```python
from build123d import *

# Parameters (mm, degrees)
F0_W      = 23
F0_H      = 16
F1_DEPTH  = 21
F2_R      = 2.5
F3_W      = 9.25
F3_H      = 5.75
F4_DEPTH  = 18
F5_R      = 1.5
F6_W      = 2
F6_H      = 12
F7_DEPTH  = 1.5
F8_W      = 2
F8_H      = 12
F9_DEPTH  = 1.5
F10_W     = 2
F10_H     = 12
F11_DEPTH = 1.5
F14_DEPTH = 3.5
F16_DEPTH = 1
F18_W     = 7.25
F18_H     = 1.5
F17_W     = 7.25
F17_H     = 1.5
F19_DEPTH = 0.5
F20_R     = 1.5
F21_DEPTH = 13


with BuildPart() as f1:
    # F0 (on Top) → F1 (new body)
    with BuildSketch(Plane.XY):
        Rectangle(F0_W, F0_H)
    extrude(amount=-F1_DEPTH)

    # F2
    f2_edges = [f1.edges().sort_by_distance(p)[0] for p in [
        (11.5, -8, -10.5),
        (11.5, 8, -10.5),
        (-11.5, -8, -10.5),
        (-11.5, 8, -10.5),
    ]]
    fillet(f2_edges, radius=F2_R)

    # F3 (on face) → F4 (cut)
    with BuildSketch(Plane.XY):
        with Locations((-5.375, 3.625)):
            Rectangle(F3_W, F3_H)
        with Locations((5.375, 3.625)):
            Rectangle(F3_W, F3_H)
        with Locations((5.375, -3.625)):
            Rectangle(F3_W, F3_H)
        with Locations((-5.375, -3.625)):
            Rectangle(F3_W, F3_H)
    extrude(amount=-F4_DEPTH, mode=Mode.SUBTRACT)

    # F5
    f5_edges = [f1.edges().sort_by_distance(p)[0] for p in [
        (-10, 6.5, -9),
        (-10, -6.5, -9),
        (10, -6.5, -9),
        (10, 6.5, -9),
    ]]
    fillet(f5_edges, radius=F5_R)

    # F6 (on face) → F7 (cut, through all)
    with BuildSketch(Plane.YZ.offset(0.75)):
        with Locations((-5.5, -6)):
            Rectangle(F6_W, F6_H)
        with Locations((5.5, -6)):
            Rectangle(F6_W, F6_H)
    extrude(amount=-F7_DEPTH, mode=Mode.SUBTRACT)

    # F8 (on face) + F7_face (on face) → F9 (cut, through all)
    with BuildSketch(Plane(origin=(0, 8, 0), x_dir=(-1, 0, 0), z_dir=(0, 1, 0))):
        with Locations((7.5, -6)):
            Rectangle(F8_W, F8_H)
        with Locations((-7.5, -6)):
            Rectangle(F8_W, F8_H)
    with BuildSketch(Plane(origin=(0, 6.5, -8.8181818182), x_dir=(1, 0, 0), z_dir=(0, -1, 0))):
        Polygon((8.5, 8.8181818182), (-8.5, 8.8181818182), (-8.5, -9.1818181818), (-0.75, -9.1818181818), (-0.75, -3.1818181818), (0.75, -3.1818181818), (0.75, -9.1818181818), (8.5, -9.1818181818), align=None)
    extrude(amount=-F9_DEPTH, dir=(0, 1, 0), mode=Mode.SUBTRACT)

    # F10 (on face) → F11 (cut, through all)
    with BuildSketch(Plane.XZ.offset(8)):
        with Locations((-7.5, -6)):
            Rectangle(F10_W, F10_H)
        with Locations((7.5, -6)):
            Rectangle(F10_W, F10_H)
    extrude(amount=-F11_DEPTH, mode=Mode.SUBTRACT)

    # F13 (on face) → F14 (join)
    with BuildSketch(Plane.XY):
        with BuildLine():
            Line((-11.5, 5), (-10, 5))
            ThreePointArc((-10, 5), (-9.5606601718, 6.0606601718), (-8.5, 6.5))
            Line((-8.5, 6.5), (-8.5, 8))
            Line((-8.5, 8), (-9, 8))
            ThreePointArc((-9, 8), (-10.767766953, 7.267766953), (-11.5, 5.5))
            Line((-11.5, 5.5), (-11.5, 5))
        make_face()
        with BuildLine():
            Line((-10, -5), (-11.5, -5))
            Line((-11.5, -5), (-11.5, -5.5))
            ThreePointArc((-11.5, -5.5), (-10.767766953, -7.267766953), (-9, -8))
            Line((-9, -8), (-8.5, -8))
            Line((-8.5, -8), (-8.5, -6.5))
            ThreePointArc((-8.5, -6.5), (-9.5606601718, -6.0606601718), (-10, -5))
        make_face()
        with BuildLine():
            Line((11.5, -5), (10, -5))
            ThreePointArc((10, -5), (9.5606601718, -6.0606601718), (8.5, -6.5))
            Line((8.5, -6.5), (8.5, -8))
            Line((8.5, -8), (9, -8))
            ThreePointArc((9, -8), (10.767766953, -7.267766953), (11.5, -5.5))
            Line((11.5, -5.5), (11.5, -5))
        make_face()
        with BuildLine():
            ThreePointArc((8.5, 6.5), (9.5606601718, 6.0606601718), (10, 5))
            Line((10, 5), (11.5, 5))
            Line((11.5, 5), (11.5, 5.5))
            ThreePointArc((11.5, 5.5), (10.767766953, 7.267766953), (9, 8))
            Line((9, 8), (8.5, 8))
            Line((8.5, 8), (8.5, 6.5))
        make_face()
    extrude(amount=F14_DEPTH)

    # F15 (on face) → F16 (join)
    with BuildSketch(Plane.XY):
        Polygon((-0.75, 0.75), (-2.75, 0.75), (-2.75, -0.75), (-0.75, -0.75), (-0.75, -2.625), (0.75, -2.625), (0.75, -0.75), (2.75, -0.75), (2.75, 0.75), (0.75, 0.75), (0.75, 2.625), (-0.75, 2.625), align=None)
    extrude(amount=F16_DEPTH)

    # F18 (on face) + F17 (on face) → F19 (join)
    with BuildSketch(Plane.XY):
        with Locations((-6.375, 0)):
            Rectangle(F18_W, F18_H)
    with BuildSketch(Plane.XY):
        with Locations((6.375, 0)):
            Rectangle(F17_W, F17_H)
    extrude(amount=F19_DEPTH)

    # F20
    f20_edges = [f1.edges().sort_by_distance(p)[0] for p in [
        (11.5, 0, -21),
        (10.767767, 7.267767, -21),
        (0, 8, -21),
        (-10.767767, 7.267767, -21),
        (-11.5, 0, -21),
        (-10.767767, -7.267767, -21),
        (0, -8, -21),
        (10.767767, -7.267767, -21),
    ]]
    fillet(f20_edges, radius=F20_R)

    # F12 (on face) → F21 (join, through all)
    with BuildSketch(Plane(origin=(-6.5, 0, 0), x_dir=(0, -1, 0), z_dir=(-1, 0, 0))):
        Polygon((-8, -2), (-8, 0), (-10, -2), align=None)
        Polygon((8, -2), (10, -2), (8, 0), align=None)
    extrude(amount=-F21_DEPTH)


solid = f1.part
```
CAD build for the part. Positions are in the model's coordinates, mm. A direction names the side the tool comes from. Coordinates: 2 decimals unless noted, no trailing zeros. Write each loop counter-clockwise with the first axis right and the second up, starting at its lowest first coordinate (ties: lowest second). Pieces come first, ordered by that corner, then holes. Notation, with made-up numbers: (64, -20.75) -> (111, -20.75) arc R16 ccw to (111, -0.75) -> close; hole circle Ø2 at (65, -9.75). An arc over 180 degrees is marked (long way). Use CSV: the item, a comma, the result in double quotes. Start each with the question number.
Item 1: Two-plate mould, pull along X, no slides. Class faces 4 (the flat face through (-5, -0.75, -9)), 5 (the cylindrical face through (-0.13, 7.55, -20.57)): +X half, -X half, draft (parallel to the pull), parting line (faces both ways), or undercut.
Item 2: Tool access for faces 1 (the flat face through (8.5, -7, -4)), 2 (the flat face through (0, -4.5, -6)), 3 (the flat face through (0, 2.625, 0.5)): list every direction of +Z, -Z, +X, -X, +Y, -Y with a clear straight run to the whole face (end or side of a thin tool).
Item 3: Wall check: probe 1 along Y at (x, z) = (4, -10.75); probe 2 along X at (y, z) = (4.25, -0.5); probe 3 along X at (y, z) = (4.75, -10). Give the ranges that are in metal, low to high.
Item 4: Band-saw the part on A-A, the plane z = -15.75. Write the cut outline in (x, y).
Item 5: Band-saw the part on B-B, the plane y = 3.25. Write the cut outline in (x, z).
Item 6: Band-saw the part on C-C, the plane x = -1.75. Write the cut outline in (y, z).
Item 7: Drop flat-ended pins along their axis: P1, Ø6.5, axis at x = 3.5, y = 3.5, coming from the +Z side; P2, Ø0.8, axis at x = -8, y = 0, coming from the +Z side; P3, Ø2, axis at x = -6.5, z = -18, coming from the +Y side. Give the stop position or say it passes through.
Item 8: Band-saw the part on D-D, the plane z = -7.25. Give the number of separate pieces and of enclosed holes in the cut face, plus the area to 3 significant figures.
Response values:
1,face 4,"undercut"
1,face 5,"draft"
2,face 1,"+Z, -Y"
2,face 2,"+Z"
2,face 3,"+Z, +X, -X, +Y"
3,probe 1,"y = -8 to -6.5, -0.75 to 0.75, 6.5 to 8"
3,probe 2,"x = -11.5 to -10, -0.75 to 0.75, 10 to 11.5"
3,probe 3,"x = -11.5 to -10, 10 to 11.5"
4,outline,"(-11.5, -5.5) arc R2.5 ccw to (-9, -8) -> (9, -8) arc R2.5 ccw to (11.5, -5.5) -> (11.5, 5.5) arc R2.5 ccw to (9, 8) -> (-9, 8) arc R2.5 ccw to (-11.5, 5.5) -> close; hole (-10, -5) arc R1.5 ccw to (-8.5, -6.5) -> (-0.75, -6.5) -> (-0.75, -0.75) -> (-10, -0.75) -> close; hole (-10, 0.75) -> (-0.75, 0.75) -> (-0.75, 6.5) -> (-8.5, 6.5) arc R1.5 ccw to (-10, 5) -> close; hole (0.75, -6.5) -> (8.5, -6.5) arc R1.5 ccw to (10, -5) -> (10, -0.75) -> (0.75, -0.75) -> close; hole (0.75, 0.75) -> (10, 0.75) -> (10, 5) arc R1.5 ccw to (8.5, 6.5) -> (0.75, 6.5) -> close"
5,outline,"(-11.5, -19.5) arc R1.5 ccw to (-10, -21) -> (10, -21) arc R1.5 ccw to (11.5, -19.5) -> (11.5, 0) -> (10, 0) -> (10, -18) -> (0.75, -18) -> (0.75, 0) -> (-0.75, 0) -> (-0.75, -18) -> (-10, -18) -> (-10, 0) -> (-11.5, 0) -> close"
6,outline,"(-10, -2) -> (-8, -2) -> (-8, -19.5) arc R1.5 ccw to (-6.5, -21) -> (6.5, -21) arc R1.5 ccw to (8, -19.5) -> (8, -2) -> (10, -2) -> (8, 0) -> (6.5, 0) -> (6.5, -18) -> (0.75, -18) -> (0.75, 1) -> (-0.75, 1) -> (-0.75, -18) -> (-6.5, -18) -> (-6.5, 0) -> (-8, 0) -> close"
7,P1,"stops at z = 1"
7,P2,"stops at z = 0.5"
7,P3,"stops at y = 8"
8,separate pieces,"3"
8,enclosed holes,"0"
8,area,"134 mm2"
